Geometry check sheet. Reference: the model listing, model coordinates, mm. A direction names the side the tool comes from. Coordinates: 2 decimals unless noted, no trailing zeros. Write each loop counter-clockwise with the first axis right and the second up, starting at its lowest first coordinate (ties: lowest second). Pieces come first, ordered by that corner, then holes.
from build123d import *

# Parameters (mm, degrees)
FILLET1_R          = 2.54
SKETCH2_R          = 6.0325
CUT_EXTRUDE1_DEPTH = 2.54
FILLET2_R          = 2.54


# Some blends are built 0.0001 mm under size
with BuildPart() as part:
    # Sketch1 → Base-Revolve (revolve)
    with BuildSketch(Plane.XY, mode=Mode.PRIVATE) as base_revolve_sk:
        with BuildLine():
            ThreePointArc((11.1125, 12.7), (6.622371939, 10.840128061), (4.7625, 6.35))
            Line((4.7625, 6.35), (3.175, 6.35))
            Line((3.175, 6.35), (3.175, 0))
            Line((3.175, 0), (0, 0))
            Line((0, 0), (0, 22.225))
            Line((0, 22.225), (11.1125, 22.225))
            Line((11.1125, 22.225), (11.1125, 12.7))
        make_face()
    revolve(base_revolve_sk.sketch.rotate(Axis((0, 0, 0), (0, 1, 0)), 90), axis=Axis((0, 0, 0), (0, 1, 0)))

    # Fillet1
    # the kernel refuses this fillet: 2.54 mm, written as the material it takes off along each edge
    with BuildSketch(Plane(origin=(0, 6.35, 0), x_dir=(0, 0, -1), z_dir=(1, 0, 0))) as fillet1_piece_1:
        with BuildLine():
            CenterArc((2.57175, 2.467324348), FILLET1_R, 283.739035174, 60.14756783)
            Line((3.175, 0), (3.187065, -0.049346487))
            ThreePointArc((3.187065, -0.049346487), (3.96875, -0.0508), (4.7625, -0.0508))
            Line((4.7625, -0.0508), (4.8133, 0))
            ThreePointArc((4.8133, 0), (4.875473976, 0.882851637), (5.060768571, 1.748275538))
            Line((5.060768571, 1.748275538), (5.011964286, 1.762374534))
        make_face()
    revolve(axis=Axis((0, 6.35, 0), (0, 1, 0)), mode=Mode.SUBTRACT)
    with BuildSketch(Plane(origin=(0, 22.225, 0), x_dir=(0, 0, -1), z_dir=(1, 0, 0))) as fillet1_piece_2:
        with BuildLine():
            CenterArc((11.1125 - FILLET1_R, -FILLET1_R), FILLET1_R, 0, 90)
            Line((11.1125, -FILLET1_R), (11.1125 + FILLET1_R * 0.02, -FILLET1_R))
            Line((11.1125 + FILLET1_R * 0.02, -FILLET1_R), (11.1125 + FILLET1_R * 0.02, FILLET1_R * 0.02))
            Line((11.1125 + FILLET1_R * 0.02, FILLET1_R * 0.02), (11.1125 - FILLET1_R, FILLET1_R * 0.02))
            Line((11.1125 - FILLET1_R, FILLET1_R * 0.02), (11.1125 - FILLET1_R, 0))
        make_face()
    revolve(axis=Axis((0, 22.225, 0), (0, 1, 0)), mode=Mode.SUBTRACT)
    with BuildSketch(Plane(origin=(0, 12.7, 0), x_dir=(0, 0, -1), z_dir=(1, 0, 0))) as fillet1_piece_3:
        with BuildLine():
            CenterArc((8.5725, 2.169418994), FILLET1_R, 286.601549599, 73.398450401)
            Line((11.1125, 2.169418994), (11.1633, 2.169418994))
            Line((11.1633, 2.169418994), (11.1633, 0))
            Line((11.1633, 0), (11.1125, -0.0508))
            ThreePointArc((11.1125, -0.0508), (10.203087128, -0.116791447), (9.312728571, -0.313383113))
            Line((9.312728571, -0.313383113), (9.298214286, -0.264700718))
        make_face()
    revolve(axis=Axis((0, 12.7, 0), (0, 1, 0)), mode=Mode.SUBTRACT)

    # Sketch2 → Cut-Extrude1 (cut)
    with BuildSketch(Plane(origin=(0, 22.225, 0), x_dir=(1, 0, 0), z_dir=(0, 1, 0))):
        with Locations(Location((0, 0, 0), (0, 0, 270))):
            Circle(SKETCH2_R)
    extrude(amount=-CUT_EXTRUDE1_DEPTH, mode=Mode.SUBTRACT)

    # Fillet2
    fillet2_edges = [part.edges().sort_by_distance(p)[0] for p in [
        (0, 19.685, -6.0325),
    ]]
    fillet(fillet2_edges, radius=FILLET2_R - 0.0001)  # a hair under: the kernel refuses the full size


solid = part.part
1. Sectioned sample at C-C, the plane y = 10. Record the boundary of the cut face in (x, z), and give its area (3 significant figures).
Computed values:
outline: circle Ø11.83 at (0, 0)
area: 110 mm2
2. Draft check along X on faces 1 (the cylindrical face through (-7.5, 17.2, 8.2)), 2 (the flat face through (-6, 22.225, 2)), 3 (the flat face through (0, 19.685, 0)). Enter one of: released by +X, released by -X, zero draft, split by the parting line, or undercut.
Computed values:
face 1: split by the parting line
face 2: zero draft
face 3: undercut
3. Gauge pin test, flat ends, axial feed: pin 1 Ø6 at (x, y) = (4, 17) entering from -Z; pin 2 Ø3 at (x, z) = (-1, -8) entering from -Y; pin 3 Ø4 at (x, y) = (2.5, 15.5) entering from +Z; pin 4 Ø3 at (x, z) = (-0.5, 3) entering from -Y. Record the tip position at first contact, or that the pin passes through.
Computed values:
pin 1: stops at z = -11.07
pin 2: stops at y = 10.78
pin 3: stops at z = 11.1
pin 4: stops at y = 0
4. Thickness scan on line 1 along Y through (x, z) = (-0.25, 0) (3 decimals); line 2 along Y through (x, z) = (-7, 6.25); line 3 along X through (y, z) = (20.25, 4). Record the ranges inside material, lowest first.
Computed values:
line 1: y = 0 to 19.685
line 2: y = 12.46 to 22.09
line 3: x = -10.3 to -3.15, 3.15 to 10.3
5. Access from +Z, -Z, +X, -X, +Y, -Y to the whole of each face (thin tool, end or side, straight path). Record for faces 4 (the flat face through (0, 0, 0)), 5 (the cylindrical face through (1.93, 3.13, 2.52)).
Computed values:
face 4: +Z, -Z, +X, -X, -Y
face 5: -Y
